The listing builds one solid part. Answer for the finished solid, in the listing's coordinates (mm). A direction names the side the tool comes from. Round coordinates to 2 decimals unless told otherwise and drop trailing zeros. Loops run counter-clockwise (first coordinate to the right, second up) from the corner with the lowest first, then second, coordinate; pieces in that order, holes last. Notation, with made-up numbers: (68, 55) -> (84, 55) arc R20 cw to (84, 84) -> close; hole circle Ø10 at (21, 62). An arc over 180 degrees is marked (long way). Answer in a Markdown table with one row per item. Add a question column.
Autodesk Inventor part; units mm, degrees
ref_plane "Work Plane1" through (15, 4, 130) normal (0.5, 0.866, 0) x (0, 0, -1)
ref_plane "YZ Plane" through (0, 0, 0) normal (1, 0, 0) x (0, 1, 0)
ref_plane "XZ Plane" through (0, 0, 0) normal (0, 1, 0) x (-1, 0, 0)
sketch "Sketch1" plane through (0, 0, 0) normal (0, 1, 0) x (-1, 0, 0)
  line L0 (-15, 0) -> (-15, 130)
  line L1 (-10, 0) -> (-10, 4)
  line L2 (-15, 4) -> (-10, 4)
  line L3 (-5, 0) -> (-10, 0)
  line L4 (-5, 0) -> (-5, 4)
  line L5 (-5, 4) -> (0, 4)
  line L6 (0, 0) -> (0, 4)
  line L7 (5, 0) -> (0, 0)
  line L8 (5, 0) -> (5, 4)
  line L9 (5, 4) -> (10, 4)
  line L10 (10, 0) -> (10, 4)
  line L11 (15, 0) -> (10, 0)
  line L12 (15, 0) -> (15, 4)
  line L13 (15, 4) -> (20, 4)
  line L14 (25, 0) -> (20, 0)
  line L15 (20, 0) -> (20, 4)
  line L16 (25, 0) -> (25, 4)
  line L17 (25, 4) -> (32, 4)
  line L18 (32, 0) -> (32, 4)
  line L19 (36.6188, 0) -> (32, 0)
  line L20 (36.6188, 0) -> (36.6188, 4)
  line L21 (36.6188, 4) -> (36.6188, 126)
  line L22 (36.6188, 126) -> (36.6188, 130)
  line L23 (32, 130) -> (36.6188, 130)
  line L24 (32, 126) -> (32, 130)
  line L25 (32, 126) -> (25, 126)
  line L26 (25, 126) -> (25, 130)
  line L27 (25, 130) -> (20, 130)
  line L28 (20, 126) -> (20, 130)
  line L29 (20, 126) -> (15, 126)
  line L30 (15, 126) -> (15, 130)
  line L31 (15, 130) -> (10, 130)
  line L32 (10, 126) -> (10, 130)
  line L33 (10, 126) -> (5, 126)
  line L34 (5, 126) -> (5, 130)
  line L35 (5, 130) -> (0, 130)
  line L36 (0, 126) -> (0, 130)
  line L37 (0, 126) -> (-5, 126)
  line L38 (-5, 126) -> (-5, 130)
  line L39 (-5, 130) -> (-10, 130)
  line L40 (-10, 126) -> (-10, 130)
  line L41 (-10, 126) -> (-15, 126)
extrude "Extrusion1" add sketch "Sketch1" along normal blind 4
ref_plane "Work Plane1" through (15, 4, 130) normal (0.5, 0.866, 0) x (0, 0, -1)
sketch "Sketch5" plane through (0, 4, 0) normal (0, 1, 0) x (1, 0, 0)
  line L0 (10, 0) -> (5, 0)
  line L1 (5, 0) -> (5, -4)
  line L2 (5, -4) -> (0, -4)
  line L3 (0, -4) -> (0, 0)
  line L4 (0, 0) -> (-5, 0)
  line L5 (-5, 0) -> (-5, -4)
  line L6 (-5, -4) -> (-10, -4)
  line L7 (-10, -4) -> (-10, 0)
  line L8 (-10, 0) -> (-15, 0)
  line L9 (-15, 0) -> (-15, -4)
  line L10 (-15, -4) -> (-20, -4)
  line L11 (-20, -4) -> (-20, 0)
  line L12 (-20, 0) -> (-25, 0)
  line L13 (-25, 0) -> (-25, -4)
  line L14 (-25, -4) -> (-32, -4)
  line L15 (-32, -4) -> (-32, 0)
  line L16 (-32, 0) -> (-36.6188, 0)
  line L17 (-36.6188, 0) -> (-36.6188, -130)
  line L18 (-36.6188, -130) -> (-32, -130)
  line L19 (-32, -130) -> (-32, -126)
  line L20 (-32, -126) -> (-25, -126)
  line L21 (-25, -126) -> (-25, -130)
  line L22 (-25, -130) -> (-20, -130)
  line L23 (-20, -130) -> (-20, -126)
  line L24 (-20, -126) -> (-15, -126)
  line L25 (-15, -126) -> (-15, -130)
  line L26 (-15, -130) -> (-10, -130)
  line L27 (-10, -130) -> (-10, -126)
  line L28 (-10, -126) -> (-5, -126)
  line L29 (-5, -126) -> (-5, -130)
  line L30 (-5, -130) -> (0, -130)
  line L31 (0, -130) -> (0, -126)
  line L32 (0, -126) -> (5, -126)
  line L33 (5, -126) -> (5, -130)
  line L34 (5, -130) -> (10, -130)
  line L35 (10, -130) -> (10, -126)
  line L36 (10, -126) -> (15, -126)
  line L37 (15, -126) -> (15, -4)
  line L38 (15, -4) -> (10, -4)
  line L39 (10, -4) -> (10, 0)
sketch "Sketch6" plane through (0, 4, 0) normal (0, 1, 0) x (1, 0, 0)
  circle A0 centre (-9.6772, -26.5655) radius 17
  circle A1 centre (-9.6772, -64.9437) radius 17
  circle A2 centre (-9.6772, -103.3775) radius 17
  point P0 (0, 0)
  dimension "d16" = 34
  dimension "d17" = 34
  dimension "d18" = 34
extrude "Extrusion4" cut sketch "Sketch6" against normal blind 5.5
properties part number "Angle Cover"
Item 1: Section A-A, the plane z = 68 is taken. Write down the section's boundary in (x, y).
Item 2: The mould has two halves that part along Z. Classify faces 6 (the flat face through (10, 2, 128)), 7 (the cylindrical face through (6.54, 2.03, 21.46)), 8 (the flat face through (-17, 2, 4)), 9 (the cylindrical face through (-0.54, 2.03, 89.04)): +Z half, -Z half, draft (parallel to the pull), parting line (faces both ways), or undercut.
Item 3: Section B-B, the plane x = -22 is taken. Write down the section's boundary in (y, z).
Item 4: Section D-D, the plane y = 2.05 is taken. Give the number of separate pieces and of enclosed holes in the cut face, and give its area (3 significant figures).
Item 5: For faces 1 (the flat face through (-13, 2, 0)), 2 (the flat face through (10, 2, 2)), 3 (the flat face through (5, 2, 128)), 4 (the flat face through (-32, 2, 2)), 5 (the flat face through (-28, 4, 66)), determine the directions among +Z, -Z, +X, -X, +Y, -Y from which every point of the face is accessible in a straight line to the end or side of a thin tool.
Item 6: Consider L1, parallel to Z at x = -3, y = 3.15; L2, parallel to Z at x = -17, y = 2.5; L3, parallel to Z at x = -27.5, y = 1.5. Determine where each line is inside the solid, lowest interval first. Write a range as from..to.
Item 7: Flat-ended cylindrical pins translate along their axes: P1, Ø2, axis at x = -18.5, y = 1, coming from the +Z side; P2, Ø1.2, axis at x = 13, y = 1.5, coming from the -Z side; P3, Ø5, axis at x = -1, z = 45, coming from the -Y side; P4, Ø1.2, axis at y = 2.5, z = 127.5, coming from the +X side. Find the tip coordinate at first contact, or state that the pin passes through.
Item 8: Section C-C, the plane z = 106 is taken. Write down the section's boundary in (x, y).
Here are the results:
| question | item | result |
|---|---|---|
| 1 | outline | (-36.62, 0) -> (-26.4, 0) -> (-26.4, 4) -> (-36.62, 4) -> close; (7.05, 0) -> (15, 0) -> (15, 4) -> (7.05, 4) -> close |
| 2 | face 6 | draft |
| 2 | face 7 | undercut |
| 2 | face 8 | -Z half |
| 2 | face 9 | undercut |
| 3 | outline | (0, 0) -> (4, 0) -> (4, 14.85) -> (0, 14.85) -> close; (0, 38.28) -> (4, 38.28) -> (4, 53.23) -> (0, 53.23) -> close; (0, 76.65) -> (4, 76.65) -> (4, 91.67) -> (0, 91.67) -> close; (0, 115.09) -> (4, 115.09) -> (4, 130) -> (0, 130) -> close |
| 4 | separate pieces | 1 |
| 4 | enclosed holes | 3 |
| 4 | area | 3,770 mm² |
| 5 | face 1 | -Z, +X, -X, +Y, -Y |
| 5 | face 2 | -Z, +X, +Y, -Y |
| 5 | face 3 | +Z, +Y, -Y |
| 5 | face 4 | -Z, +Y, -Y |
| 5 | face 5 | +Z, -Z, +X, -X, +Y |
| 6 | L1 | z = 0..10.93, 42.2..49.31, 80.58..87.74, 119.01..130 |
| 6 | L2 | z = 4..11.22, 41.91..49.6, 80.29..88.04, 118.72..126 |
| 6 | L3 | z = 4..126 |
| 7 | P1 | stops at z = 126 |
| 7 | P2 | stops at z = 4 |
| 7 | P3 | stops at y = 0 |
| 7 | P4 | stops at x = 10 |
| 8 | outline | (-36.62, 0) -> (-26.47, 0) -> (-26.47, 4) -> (-36.62, 4) -> close; (7.12, 0) -> (15, 0) -> (15, 4) -> (7.12, 4) -> close |
